from build123d import *

# Parameters (mm, degrees)
F1_DEPTH      = 1524
F2_R          = 1.5875
F3_DEPTH      = 1524.001
F4_W          = 0.3175
F4_H          = 44.45
F5_DEPTH      = 193.3445428183
F5_DEPTH_BACK = 192.6822115509


with BuildPart() as f1:
    # F0 (on Right) → F1 (new body)
    with BuildSketch(Plane.YZ):
        with BuildLine():
            ThreePointArc((-193.675, 57.15), (-184.8763020632, 28.575), (-193.675, 0))
            Line((-193.675, 0), (193.675, 0))
            ThreePointArc((193.675, 0), (187.5626801821, 28.575), (193.675, 57.15))
            Line((193.675, 57.15), (186.7733895925, 57.15))
            ThreePointArc((186.7733895925, 57.15), (181.2871488449, 31.94300811), (184.5258543835, 6.35))
            Line((184.5258543835, 6.35), (-183.0248835163, 6.35))
            ThreePointArc((-183.0248835163, 6.35), (-178.6364166438, 32.1209796041), (-186.1829502369, 57.15))
            Line((-186.1829502369, 57.15), (-193.675, 57.15))
        make_face()
    extrude(amount=-F1_DEPTH)

    # F2 (on face) → F3 (cut, through all)
    with BuildSketch(Plane.YZ):
        with Locations((190.5, 53.975)):
            Circle(F2_R)
        with Locations((190.5, 3.175)):
            Circle(F2_R)
    extrude(amount=-F3_DEPTH, mode=Mode.SUBTRACT)

    # F4 (on Front) → F5 (cut, two sides)
    with BuildSketch(Plane.XZ) as f5_sk:
        with Locations((-50.95875, 31.75)):
            Rectangle(F4_W, F4_H)
        with Locations((-152.55875, 31.75)):
            Rectangle(F4_W, F4_H)
        with Locations((-254.15875, 31.75)):
            Rectangle(F4_W, F4_H)
        with Locations((-355.75875, 31.75)):
            Rectangle(F4_W, F4_H)
        with Locations((-457.35875, 31.75)):
            Rectangle(F4_W, F4_H)
        with Locations((-558.95875, 31.75)):
            Rectangle(F4_W, F4_H)
        with Locations((-660.55875, 31.75)):
            Rectangle(F4_W, F4_H)
        with Locations((-762.15875, 31.75)):
            Rectangle(F4_W, F4_H)
        with Locations((-863.75875, 31.75)):
            Rectangle(F4_W, F4_H)
        with Locations((-965.35875, 31.75)):
            Rectangle(F4_W, F4_H)
        with Locations((-1066.95875, 31.75)):
            Rectangle(F4_W, F4_H)
        with Locations((-1168.55875, 31.75)):
            Rectangle(F4_W, F4_H)
        with Locations((-1270.15875, 31.75)):
            Rectangle(F4_W, F4_H)
        with Locations((-1371.75875, 31.75)):
            Rectangle(F4_W, F4_H)
        with Locations((-1473.35875, 31.75)):
            Rectangle(F4_W, F4_H)
    extrude(amount=-F5_DEPTH, mode=Mode.SUBTRACT)
    extrude(f5_sk.sketch, amount=F5_DEPTH_BACK, mode=Mode.SUBTRACT)


solid = f1.part
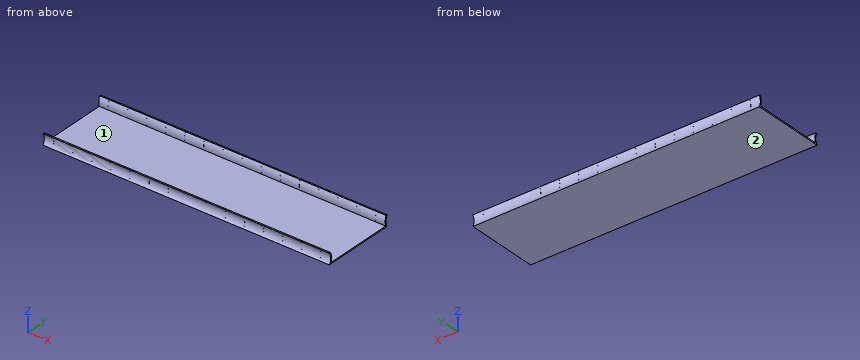
Geometry check sheet. Reference: the model listing, model coordinates, mm. Face numbers are marked on the shaded views. Round coordinates to 2 decimals unless told otherwise and drop trailing zeros. Order: outer loops, then holes, each group sorted by start corner. A loop starts at its lowest first (then second) coordinate and runs counter-clockwise, first axis right, second up. Notation, with made-up numbers: M -25,51 L 32,51 A20 cw 32,73 Z; hole C -9.5,33 d10. An arc over 180 degrees is marked long. Write each question's results on one line, items separated by ' | '. Start each with the question number.
1. Cross-section at A-A on x = -520.5. Give the number of separate pieces and of enclosed holes in the cut face, plus the area to 3 significant figures.
2. Material ranges on L1, parallel to Y at x = -682, z = 25; L2, parallel to Z at x = -1461.5, y = 32.5; L3, parallel to Y at x = -638, z = 15.5, recorded low to high. Write a range as from..to.
3. Go/stop test with flat-tipped pins: P1, Ø1, axis at x = -569.5, z = 10.5, coming from the -Y side; P2, Ø5, axis at x = -672.5, z = 49, coming from the +Y side; P3, Ø10, axis at x = -1176, y = 10.5, coming from the +Z side. Record where each tip stops, or that it passes through.
4. Cross-section at C-C on y = -136.5. Record the boundary of the cut face in (x, z).
5. Draft check along Y on the marked faces 1 and 2. Enter one of: pulls with the +Y half, pulls with the -Y half, needs draft (parallel to the pull), parting line crosses it, or undercut.
Resolved:
1) separate pieces: 1 | enclosed holes: 2 | area: 3,090 mm2
2) L1: -185..-178.64, 181.3..187.65 | L2: 0..6.35 | L3: -186.59..-180.04, 182.34..188.8
3) P1: y = -188.39 | P2: y = 191.43 | P3: z = 6.35
4) outline: M -1524,0 L 0,0 L 0,6.35 L -1524,6.35 Z
5) face 1: undercut | face 2: needs draft
